```python
from build123d import *

# Parameters (mm, degrees)
BOSS_EXTRU_1_DEPTH = 5


with BuildPart() as part:
    # Esquisse1 → Boss.-Extru.1 (new body)
    with BuildSketch(Plane.XY):
        Polygon((-30, 188), (-45, 188), (-89, 188), (-104, 188), (-104, 193), (-109, 193), (-109, 188), (-114, 188), (-119, 188), (-119, 193), (-124, 193), (-124, 188), (-144, 188), (-144, 193), (-149, 193), (-149, 188), (-154, 188), (-159, 188), (-159, 193), (-164, 193), (-164, 188), (-179, 188), (-179, 0), (-164, 0), (-164, -5), (-159, -5), (-159, 0), (-154, 0), (-149, 0), (-149, -5), (-144, -5), (-144, 0), (-124, 0), (-124, -5), (-119, -5), (-119, 0), (-114, 0), (-109, 0), (-109, -5), (-104, -5), (-104, 0), (-89, 0), (-45, 0), (-30, 0), (-30, -5), (-25, -5), (-25, 0), (-20, 0), (-15, 0), (-15, -5), (-10, -5), (-10, 0), (10, 0), (10, -5), (15, -5), (15, 0), (20, 0), (25, 0), (25, -5), (30, -5), (30, 0), (45, 0), (45, 188), (30, 188), (30, 193), (25, 193), (25, 188), (20, 188), (15, 188), (15, 193), (10, 193), (10, 188), (-10, 188), (-10, 193), (-15, 193), (-15, 188), (-20, 188), (-25, 188), (-25, 193), (-30, 193), align=None)
        Polygon((-45, 125.5), (-89, 125.5), (-89, 50.5), (-67, 50.5), (-45, 50.5), align=None, mode=Mode.SUBTRACT)
    extrude(amount=BOSS_EXTRU_1_DEPTH)


solid = part.part
```
Model file for the job. Use its own axes, mm. A direction names the side the tool comes from. Give positions to 0.01 mm unless a question says otherwise; leave off trailing zeros. Write each loop counter-clockwise with the first axis right and the second up, starting at its lowest first coordinate (ties: lowest second). Pieces come first, ordered by that corner, then holes. Notation, with made-up numbers: (56, 17.5) - (74, 17.5) arc R19 ccw to (74, 23.5) - close; hole circle Ø7 at (19, -32.5). An arc over 180 degrees is marked (long way). One line per question, with ' | ' between items. Start each with the question number.
(1) Two-plate mould, pull along X, no slides. Class faces 1 (the face through (-121, 193, 2)), 2 (the face through (-154, 188, 2)), 3 (the face through (-179, 95, 2)): +X half, -X half, draft (parallel to the pull), parting line (faces both ways), or undercut.
(2) 3-axis set-ups, long thin cutter, end or side, ignore diameter. For faces 4 (the face through (-164, -2, 2)), 5 (the face through (-67, 125.5, 2)), 6 (the face through (-119, 190, 2)), 7 (the face through (38, 188, 2)), 8 (the face through (-124, -2, 2)): which of +Z, -Z, +X, -X, +Y, -Y reach the whole face in a straight line?
(3) Pin check, flat tips, straight feed: P1, Ø1.5, axis at x = 36, z = 3, coming from the +Y side; P2, Ø1.5, axis at y = -1.5, z = 1.5, coming from the +X side; P3, Ø2.5, axis at x = -173, z = 2.5, coming from the -Y side. Stop position of each tip, or through.
(4) Slice it at C-C on x = -130. Write the cut outline in (y, z), plus the area to 3 significant figures.
(5) Wall check: line 1 along X through (y, z) = (78, 1.1); line 2 along Y through (x, z) = (2, 4.45). Give the ranges that are in metal, low to high. Write a range as from..to.
(6) Slice it at A-A on x = -74. Write the cut outline in (y, z), plus the area to 3 significant figures.
(7) Slice it at B-B on y = 121. Write the cut outline in (x, z).
Results below:
1) face 1: draft | face 2: undercut | face 3: -X half
2) face 4: +Z, -Z, -X, -Y | face 5: +Z, -Z | face 6: +Z, -Z, +Y | face 7: +Z, -Z, +X, +Y | face 8: +Z, -Z, -Y
3) P1: y = 188 | P2: x = 30 | P3: y = 0
4) outline: (0, 0) - (188, 0) - (188, 5) - (0, 5) - close | area: 940 mm^2
5) line 1: -179..-89, -45..45 | line 2: 0..188
6) outline: (0, 0) - (50.5, 0) - (50.5, 5) - (0, 5) - close; (125.5, 0) - (188, 0) - (188, 5) - (125.5, 5) - close | area: 565 mm^2
7) outline: (-179, 0) - (-89, 0) - (-89, 5) - (-179, 5) - close; (-45, 0) - (45, 0) - (45, 5) - (-45, 5) - close
